Autodesk Inventor part; units mm, degrees
ref_plane "YZ Plane" through (0, 0, 0) normal (1, 0, 0) x (0, 1, 0)
ref_plane "XZ Plane" through (0, 0, 0) normal (0, 1, 0) x (-1, 0, 0)
ref_plane "XY Plane" through (0, 0, 0) normal (0, 0, 1) x (1, 0, 0)
sketch "Sketch1" plane through (0, 0, 0) normal (0, 1, 0) x (-1, 0, 0)
  circle A0 centre (0, 0) radius 1.5
  dimension "d0" = 3
extrude "Extrusion1" add sketch "Sketch1" along normal blind 1
sketch "Sketch2" plane through (0, 1, 0) normal (0, 1, 0) x (1, 0, 0)
  circle A0 centre (0, 0) radius 0.75
  dimension "d3" = 1.5
extrude "Extrusion2" add sketch "Sketch2" along normal blind 12
sketch "Sketch3" plane through (0, 0, 0) normal (0, -1, 0) x (1, 0, 0)
  line L0 (0.25, 1.5) -> (-0.25, 1.5)
  line L1 (-0.25, 1.5) -> (-0.25, -1.5)
  line L2 (-0.25, -1.5) -> (0.25, -1.5)
  line L3 (0.25, -1.5) -> (0.25, 1.5)
  line L4 (0.25, 1.5) -> (-0.25, -1.5) construction
  line L5 (-0.25, 1.5) -> (0.25, -1.5) construction
  circle A0 centre (0, 0) radius 1.5
  point P0 (0.25, -1.479)
  point P1 (0.25, 1.479)
  point P2 (-0.25, 1.479)
  point P3 (-0.25, -1.479)
  dimension "d6" = 0.5
extrude "Extrusion3" cut sketch "Sketch3" against normal blind 0.3 contours A0 L3 L1
properties part number "m1.5_bolt_12mm" material "Brass, Soft Yellow"
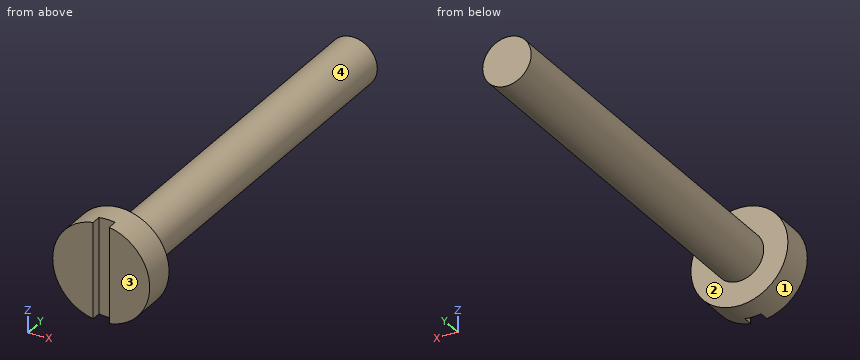
Part model, mm, in its own coordinate system. Face numbers are marked on the shaded views. A direction names the side the tool comes from. Give positions to 0.01 mm unless a question says otherwise; leave off trailing zeros. Order: outer loops, then holes, each group sorted by start corner. A loop starts at its lowest first (then second) coordinate and runs counter-clockwise, first axis right, second up. Notation, with made-up numbers: (26, 33.25) - (33, 33.25) arc R27 ccw to (33, 55.25) - close; hole circle Ø7 at (-8, 19.25). An arc over 180 degrees is marked (long way). Use a Markdown table: item, result.
1) Saw through at D-D on x = -0.6. List the corners of the cut face in (y, z), plus the area to 3 significant figures.
Checked values:
| item | result |
|---|---|
| outline | (0, -1.37) - (1, -1.37) - (1, -0.45) - (13, -0.45) - (13, 0.45) - (1, 0.45) - (1, 1.37) - (0, 1.37) - close |
| area | 13.5 mm² |
2) 3-axis set-ups, long thin cutter, end or side, ignore diameter. For the marked faces 3 and 4: which of +Z, -Z, +X, -X, +Y, -Y reach the whole face in a straight line?
Checked values:
| item | result |
|---|---|
| face 3 | +Z, -Z, +X, -X, -Y |
| face 4 | +Y |
3) Saw through at A-A on x = 0. List the corners of the cut face in (y, z).
Checked values:
| item | result |
|---|---|
| outline | (0.3, -1.5) - (1, -1.5) - (1, -0.75) - (13, -0.75) - (13, 0.75) - (1, 0.75) - (1, 1.5) - (0.3, 1.5) - close |
4) Flat gauge pin, fed straight in: P1, Ø1.5, axis at x = 0.5, y = 2.5, coming from the +Z side. Where does the tip first touch, or does it go through?
Checked values:
| item | result |
|---|---|
| P1 | z = 0.75 |
5) Saw through at C-C on y = 10.25. List the corners of the cut face in (x, z).
Checked values:
| item | result |
|---|---|
| outline | circle Ø1.5 at (0, 0) |
6) Probe L1, parallel to Y at x = 0.15, z = -0.45; L2, parallel to X at y = 1.75, z = 0.05; L3, parallel to Y at x = 1.3, z = 0.55. List the from-to ranges inside material, lowest first. Write a range as from..to.
Checked values:
| item | result |
|---|---|
| L1 | 0.3..13 |
| L2 | -0.75..0.75 |
| L3 | 0..1 |
7) Two-plate mould, pull along X, no slides. Class the marked faces 1 and 2: +X half, -X half, draft (parallel to the pull), parting line (faces both ways), or undercut.
Checked values:
| item | result |
|---|---|
| face 1 | parting line |
| face 2 | draft |
8) Saw through at B-B on z = 0. List the corners of the cut face in (x, y), plus the area to 4 significant figures.
Checked values:
| item | result |
|---|---|
| outline | (-1.5, 0) - (-0.25, 0) - (-0.25, 0.3) - (0.25, 0.3) - (0.25, 0) - (1.5, 0) - (1.5, 1) - (0.75, 1) - (0.75, 13) - (-0.75, 13) - (-0.75, 1) - (-1.5, 1) - close |
| area | 20.85 mm² |
